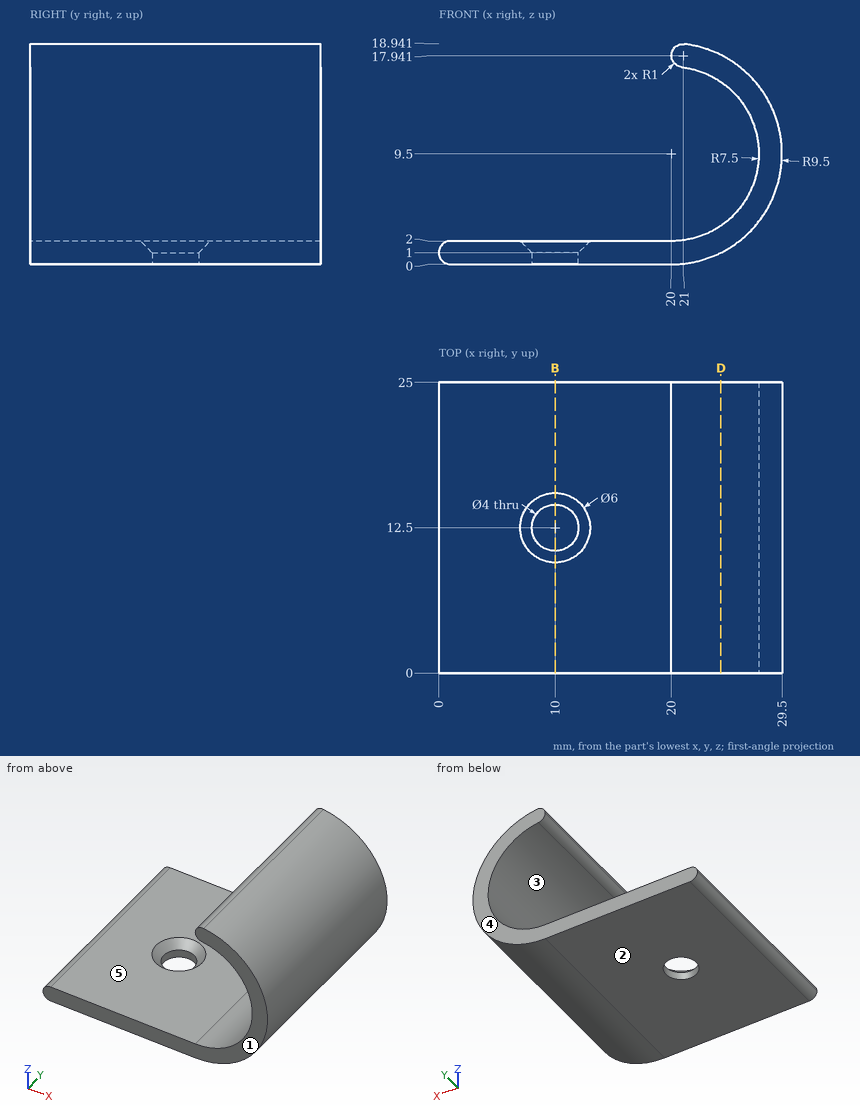
For this review, use the dimensioned drawing (mm, ordinates from the lowest corner) and the shaded views. A direction names the side the tool comes from. Coordinates: 2 decimals unless noted, no trailing zeros. Loops run counter-clockwise (first coordinate to the right, second up) from the corner with the lowest first, then second, coordinate; pieces in that order, holes last.
1. Insertion check: P1, Ø6, axis at y = 22, z = 11, coming from the -X side; P2, Ø12, axis at x = 6, y = 18, coming from the +Z side; P3, Ø1.5, axis at y = 13.5, z = 13.5, coming from the +X side. Each pin has a flat end and moves straight along its axis. Give the tip position at first contact, or say it passes through.
2. For line 1 (Y direction, x = 10, z = 0.4); line 2 (Z direction, x = 10.75, y = 4); line 3 (Z direction, x = 21.5, y = 2.5), list the stretches that pass through material, from the lowest coordinate up.
3. Add section D-D, the plane x = 24.25. Give the boundary of the cut face in (y, z).
4. For the marked faces 4 and 5, list the 3-axis set-ups (+Z, -Z, +X, -X, +Y, -Y) from which the entire face can be reached by the end or side of a thin tool; tool diameter is ignored.
5. Add section B-B, the plane x = 10. Give the boundary of the cut face in (y, z), then the cut area to 3 significant figures.
6. Mouldability with a two-part tool opening along Z and no side actions: class the marked faces 1, 2 and 3 as +Z half, -Z half, draft (parallel to the pull), parting line (faces both ways), or undercut.
Result:
1. P1: stops at x = 26
1. P2: stops at z = 2
1. P3: stops at x = 28.93
2. line 1: y = 0 to 10.5, 14.5 to 25
2. line 2: z = 0 to 2
2. line 3: z = 0.12 to 2.15, 16.85 to 18.88
3. outline: (0, 1) - (25, 1) - (25, 3.32) - (0, 3.32) - close; (0, 15.68) - (25, 15.68) - (25, 18) - (0, 18) - close
4. face 4: +Z, -Z, +X, -X, +Y
4. face 5: +Z, -X, +Y, -Y
5. outline: (0, 0) - (10.5, 0) - (10.5, 1) - (9.5, 2) - (0, 2) - close; (14.5, 0) - (25, 0) - (25, 2) - (15.5, 2) - (14.5, 1) - close
5. area: 41.0 mm2
6. face 1: draft
6. face 2: -Z half
6. face 3: undercut
